Geometry: see drawing. Coordinates: mm, zero at the bounding-box minimum. A direction names the side the tool comes from. Coordinates: 2 decimals unless noted, no trailing zeros. Loops run counter-clockwise (first coordinate to the right, second up) from the corner with the lowest first, then second, coordinate; pieces in that order, holes last. Notation, with made-up numbers: (69, 58.25) - (119, 58.25) arc R10 ccw to (119, 73.25) - close; hole circle Ø6 at (29.5, 10.25). An arc over 180 degrees is marked (long way). Use a Markdown table: item, result. Add a question column.
1. Contact query for flat-ended pins moving along their axis: P1, Ø3, axis at x = 15.5, y = 15.5, coming from the -Z side; P2, Ø8, axis at y = 15, z = 5.5, coming from the +X side; P3, Ø4, axis at y = 12, z = 13.5, coming from the +X side; P4, Ø5, axis at x = 2.5, y = 8, coming from the -Z side. Output: stop coordinate, or through.
2. Access query for the marked faces 1 and 2. Directions: +Z, -Z, +X, -X, +Y, -Y. A direction counts if a zero-diameter tool reaches every point of the face in a straight line with its end or side. Return the directions, or none.
3. Section query C-C on x = 8.5. Return the cut outline in (y, z), then the cut area to 4 significant figures.
4. Section query A-A on x = 14.5. Return the cut outline in (y, z).
5. Ray query, L1, parallel to Z at x = 14.5, y = 1.2; L2, parallel to Y at x = 14.75, z = 8. Return the intervals inside material, ascending. Write a range as [from, to].
6. Section query B-B on z = 2.5. Return the cut outline in (x, y), then the cut area to 3 significant figures.
7. Section query D-D on z = 8.5. Return the cut outline in (x, y), then the cut area to 4 significant figures.
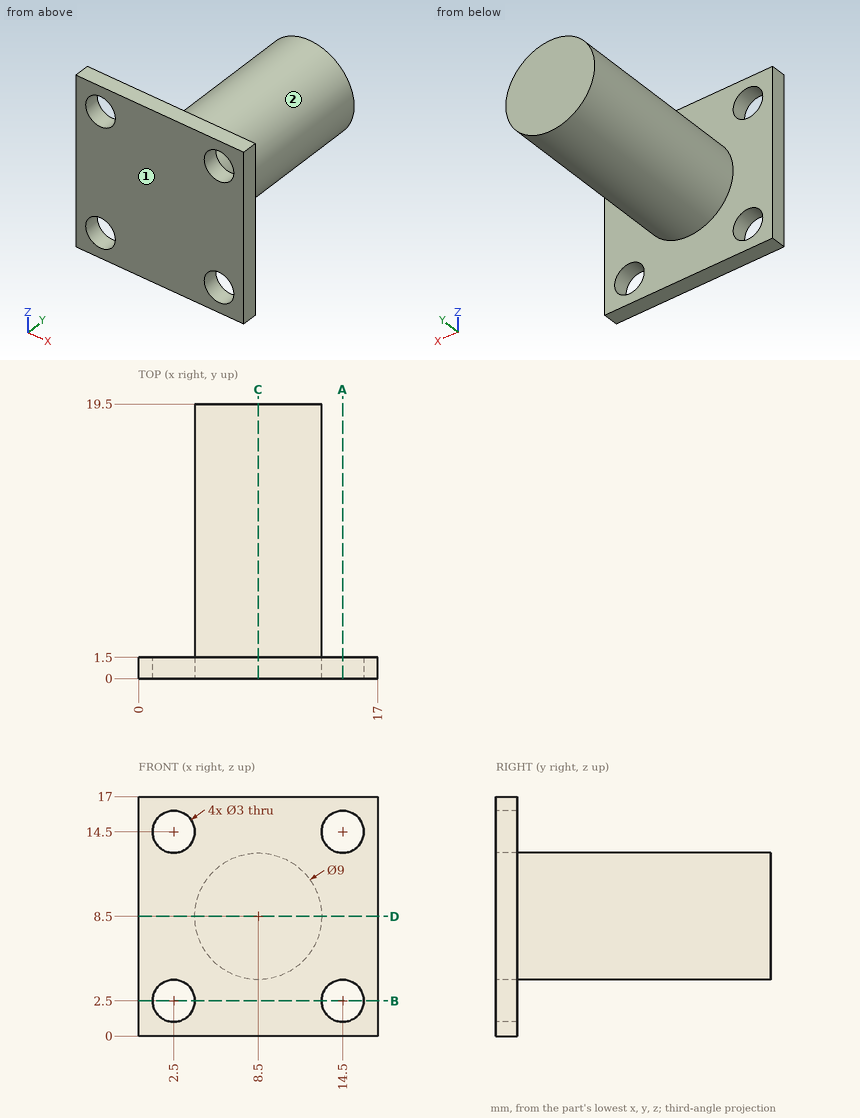
Resolved:
| question | item | result |
|---|---|---|
| 1 | P1 | through |
| 1 | P2 | x = 13 |
| 1 | P3 | x = 11.85 |
| 1 | P4 | z = 5.67 |
| 2 | face 1 | +Z, -Z, +X, -X, -Y |
| 2 | face 2 | +Y |
| 3 | outline | (0, 0) - (1.5, 0) - (1.5, 4) - (19.5, 4) - (19.5, 13) - (1.5, 13) - (1.5, 17) - (0, 17) - close |
| 3 | area | 187.5 mm² |
| 4 | outline | (0, 0) - (1.5, 0) - (1.5, 1) - (0, 1) - close; (0, 4) - (1.5, 4) - (1.5, 13) - (0, 13) - close; (0, 16) - (1.5, 16) - (1.5, 17) - (0, 17) - close |
| 5 | L1 | [0, 1], [4, 13], [16, 17] |
| 5 | L2 | [0, 1.5] |
| 6 | outline | (0, 0) - (1, 0) - (1, 1.5) - (0, 1.5) - close; (4, 0) - (13, 0) - (13, 1.5) - (4, 1.5) - close; (16, 0) - (17, 0) - (17, 1.5) - (16, 1.5) - close |
| 6 | area | 16.5 mm² |
| 7 | outline | (0, 0) - (17, 0) - (17, 1.5) - (13, 1.5) - (13, 19.5) - (4, 19.5) - (4, 1.5) - (0, 1.5) - close |
| 7 | area | 187.5 mm² |
